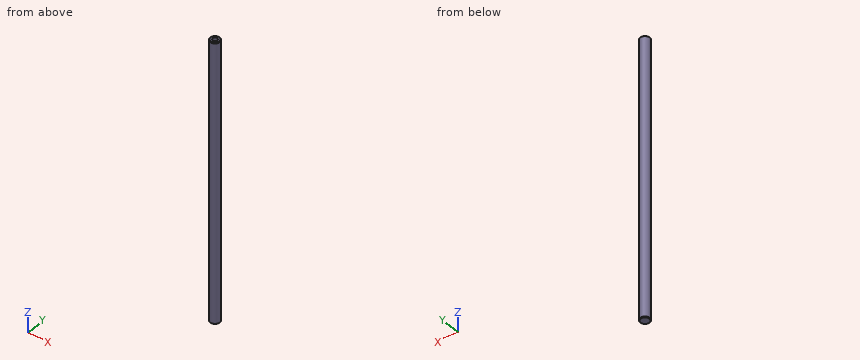
```python
from build123d import *

# Parameters (mm, degrees)
SKIZZE1_R                    = 9
BASIS_LINEAR_AUSTRAGEN_DEPTH = 267.5
FASE1_SIZE                   = 1
BOHRUNG1_D                   = 8.5
BOHRUNG1_DEPTH               = 23
BOHRUNG1_TIP                 = 2.553657631


with BuildPart() as part:
    # Skizze1 → Basis-Linear austragen (new, symmetric)
    with BuildSketch(Plane.XY):
        Circle(SKIZZE1_R)
    extrude(amount=BASIS_LINEAR_AUSTRAGEN_DEPTH, both=True)

    # Fase1
    fase1_edges = [part.edges().sort_by_distance(p)[0] for p in [
        (-9, 0, -267.5),
        (-9, 0, 267.5),
    ]]
    chamfer(fase1_edges, length=FASE1_SIZE)

    # Bohrung1
    with Locations(Plane.XY.offset(267.5)):
        with Locations((0, 0)):
            Hole(BOHRUNG1_D / 2, depth=BOHRUNG1_DEPTH)
            with Locations((0, 0, -(BOHRUNG1_DEPTH + BOHRUNG1_TIP / 2))):  # 118° drill point
                Cone(0, BOHRUNG1_D / 2, BOHRUNG1_TIP, mode=Mode.SUBTRACT)


solid = part.part
```
The listing builds one solid part. Answer for the finished solid, in the listing's coordinates (mm). Coordinates: 2 decimals unless noted, no trailing zeros. Loops run counter-clockwise (first coordinate to the right, second up) from the corner with the lowest first, then second, coordinate; pieces in that order, holes last. Notation, with made-up numbers: M 41,81.5 L 75,81.5 A22 ccw 75,94.5 Z; hole C 59.25,48.5 d4. An arc over 180 degrees is marked long. Answer as a JSON object with one key per item and string values. Group by question number.
Item 1: Section A-A (z = -51) is taken. Write down the section's boundary in (x, y).
Item 2: This flat-tipped pin is pushed along its axis until it touches: P1, Ø1.5, axis at x = -6, z = 100, coming from the +Y side. Where does it stop, or does it pass through?
Item 3: Consider L1, parallel to Y at x = 0, z = 253.5; L2, parallel to Y at x = 0.5, z = 11; L3, parallel to Y at x = -1, z = 149. Determine where each line is inside the solid, lowest interval first.
Solved:
{
 "1": {"outline": "C 0,0 d18"},
 "2": {"P1": "stops at y = 7.31"},
 "3": {"L1": "y = -9 to -4.25, 4.25 to 9", "L2": "y = -8.99 to 8.99", "L3": "y = -8.94 to 8.94"}
}
